```python
from build123d import *

# Parameters (mm, degrees)
SKETCH_2_R          = 7.1
SKETCH_2_R_2        = 6.1
EXTRUDE_1_DEPTH     = 2.2
SKETCH_2_3_R        = 9
SKETCH_2_3_R_2      = 7.1
EXTRUDE_2_DEPTH     = 4
EXTRUDE_3_DEPTH     = 4
SKETCH_4_W          = 46
SKETCH_4_H          = 28
SKETCH_4_W_2        = 38
SKETCH_4_H_2        = 21
EXTRUDE_4_DEPTH     = 4
EXTRUDE_1_2_DEPTH   = 4
DELETE_FACE_1_DEPTH = 4
FILLET_4_R          = 0.5
FILLET_5_R          = 0.4
FILLET_6_R          = 1


# Read off the part's stored shape, not the designer's step: 删除面1
with BuildPart() as part:
    # 草图2 → Extrude 1 (new body)
    with BuildSketch(Plane.XY):
        Circle(SKETCH_2_R)
        Circle(SKETCH_2_R_2, mode=Mode.SUBTRACT)
    extrude(amount=EXTRUDE_1_DEPTH)

    # 草图2<3> → 凸台-拉伸2 (add)
    with BuildSketch(Plane.XY):
        Circle(SKETCH_2_3_R)
        Circle(SKETCH_2_3_R_2, mode=Mode.SUBTRACT)
    extrude(amount=EXTRUDE_2_DEPTH)

    # 草图3 → 凸台-拉伸3 (add)
    with BuildSketch(Plane.XY):
        with BuildLine():
            Line((6, 6.708203932), (6, 9.5))
            Line((6, 9.5), (-6, 9.5))
            Line((-6, 9.5), (-6, 6.708203932))
            ThreePointArc((-6, 6.708203932), (0, 9), (6, 6.708203932))
        make_face()
        with BuildLine():
            Line((-6, -9.5), (6, -9.5))
            Line((6, -9.5), (6, -6.708203932))
            ThreePointArc((6, -6.708203932), (0, -9), (-6, -6.708203932))
            Line((-6, -6.708203932), (-6, -9.5))
        make_face()
    extrude(amount=EXTRUDE_3_DEPTH)



with BuildPart() as body_2:
    # 草图4 → 凸台-拉伸4 (new body)
    with BuildSketch(Plane.XY):
        with Locations((0, 1)):
            Rectangle(SKETCH_4_W, SKETCH_4_H)
        with Locations((0, 0.5)):
            Rectangle(SKETCH_4_W_2, SKETCH_4_H_2, mode=Mode.SUBTRACT)
    extrude(amount=EXTRUDE_4_DEPTH)


with BuildPart() as part_1:
    add(part.part)

    add(body_2.part)  # Extrude 1 2 merges body 2
    # 草图7 → Extrude 1 2 (add)
    with BuildSketch(Plane.XY):
        with BuildLine():
            ThreePointArc((19.19111663, -8.148610709), (15.188418529, -6.736776188), (10.944962783, -6.647601418))
            ThreePointArc((10.944962783, -6.647601418), (8.412688328, -7.06534444), (5.904962783, -7.611454086))
            Line((5.904962783, -7.611454086), (6.095037217, -8.388545914))
            ThreePointArc((6.095037217, -8.388545914), (8.562957594, -7.851104675), (11.055037217, -7.439992495))
            ThreePointArc((11.055037217, -7.439992495), (15.04515232, -7.523843398), (18.80888337, -8.851389291))
            Line((18.80888337, -8.851389291), (19.19111663, -8.148610709))
        make_face()
        with BuildLine():
            ThreePointArc((-18.80888337, -8.851389291), (-15.04515232, -7.523843398), (-11.055037217, -7.439992495))
            ThreePointArc((-11.055037217, -7.439992495), (-8.562957594, -7.851104675), (-6.095037217, -8.388545914))
            Line((-6.095037217, -8.388545914), (-5.904962783, -7.611454086))
            ThreePointArc((-5.904962783, -7.611454086), (-8.412688328, -7.06534444), (-10.944962783, -6.647601418))
            ThreePointArc((-10.944962783, -6.647601418), (-15.188418529, -6.736776188), (-19.19111663, -8.148610709))
            Line((-19.19111663, -8.148610709), (-18.80888337, -8.851389291))
        make_face()
        with BuildLine():
            ThreePointArc((-18.80888337, 7.148610709), (-15.04515232, 8.476156602), (-11.055037217, 8.560007505))
            ThreePointArc((-11.055037217, 8.560007505), (-8.562957594, 8.148895325), (-6.095037217, 7.611454086))
            Line((-6.095037217, 7.611454086), (-5.904962783, 8.388545914))
            ThreePointArc((-5.904962783, 8.388545914), (-8.412688328, 8.93465556), (-10.944962783, 9.352398582))
            ThreePointArc((-10.944962783, 9.352398582), (-15.188418529, 9.263223812), (-19.19111663, 7.851389291))
            Line((-19.19111663, 7.851389291), (-18.80888337, 7.148610709))
        make_face()
        with BuildLine():
            ThreePointArc((19.19111663, 7.851389291), (15.188418529, 9.263223812), (10.944962783, 9.352398582))
            ThreePointArc((10.944962783, 9.352398582), (8.412688328, 8.93465556), (5.904962783, 8.388545914))
            Line((5.904962783, 8.388545914), (6.095037217, 7.611454086))
            ThreePointArc((6.095037217, 7.611454086), (8.562957594, 8.148895325), (11.055037217, 8.560007505))
            ThreePointArc((11.055037217, 8.560007505), (15.04515232, 8.476156602), (18.80888337, 7.148610709))
            Line((18.80888337, 7.148610709), (19.19111663, 7.851389291))
        make_face()
    extrude(amount=EXTRUDE_1_2_DEPTH)

    # Delete Face 1 outline → Delete Face 1 (add)
    with BuildSketch(Plane.XY):
        with BuildLine():
            ThreePointArc((-19, 7.042506057), (-18.904671788, 7.095972847), (-18.80888337, 7.148610709))
            Line((-18.80888337, 7.148610709), (-19, 7.5))
            Line((-19, 7.5), (-19, 7.042506057))
        make_face()
        with BuildLine():
            Line((-6, 7.588108866), (-6, 8))
            Line((-6, 8), (-6.095037217, 7.611454086))
            ThreePointArc((-6.095037217, 7.611454086), (-6.047512851, 7.599804915), (-6, 7.588108866))
        make_face()
        with BuildLine():
            ThreePointArc((-19, -8.957493943), (-18.904671788, -8.904027153), (-18.80888337, -8.851389291))
            Line((-18.80888337, -8.851389291), (-19, -8.5))
            Line((-19, -8.5), (-19, -8.957493943))
        make_face()
        with BuildLine():
            Line((-6, -8.411891134), (-6, -8))
            Line((-6, -8), (-6.095037217, -8.388545914))
            ThreePointArc((-6.095037217, -8.388545914), (-6.047512851, -8.400195085), (-6, -8.411891134))
        make_face()
        with BuildLine():
            Line((6.095037217, 7.611454086), (6, 8))
            Line((6, 8), (6, 7.588108866))
            ThreePointArc((6, 7.588108866), (6.047512851, 7.599804915), (6.095037217, 7.611454086))
        make_face()
        with BuildLine():
            Line((19, 7.5), (18.80888337, 7.148610709))
            ThreePointArc((18.80888337, 7.148610709), (18.904671788, 7.095972847), (19, 7.042506057))
            Line((19, 7.042506057), (19, 7.5))
        make_face()
        with BuildLine():
            Line((6.095037217, -8.388545914), (6, -8))
            Line((6, -8), (6, -8.411891134))
            ThreePointArc((6, -8.411891134), (6.047512851, -8.400195085), (6.095037217, -8.388545914))
        make_face()
        with BuildLine():
            Line((19, -8.5), (18.80888337, -8.851389291))
            ThreePointArc((18.80888337, -8.851389291), (18.904671788, -8.904027153), (19, -8.957493943))
            Line((19, -8.957493943), (19, -8.5))
        make_face()
    extrude(amount=DELETE_FACE_1_DEPTH)

    # 圆角4
    fillet_4_edges = [part_1.edges().sort_by_distance(p)[0] for p in [
        (19, -8.046657496, 2),
        (6, -7.588305973, 2),
        (-19, -8.046657496, 2),
        (-6, -7.588305973, 2),
        (-6, 9.5, 2),
        (6, 9.5, 2),
        (6, 6.708203932, 2),
        (-6, 6.708203932, 2),
        (19, -8.957493943, 2),
        (-19, -8.957493943, 2),
        (-19, 7.042506057, 2),
        (19, 7.042506057, 2),
        (6, -6.708203932, 2),
        (-6, -6.708203932, 2),
        (-19, 7.953342504, 2),
        (19, 7.953342504, 2),
    ]]
    fillet(fillet_4_edges, radius=FILLET_4_R)

    # 圆角5
    fillet_5_edges = [part_1.edges().sort_by_distance(p)[0] for p in [
        (6, -8.411891134, 2),
        (-6, -8.411891134, 2),
        (-6, 7.588108866, 2),
        (6, 7.588108866, 2),
        (-6, -9.5, 2),
        (6, -9.5, 2),
        (-6, 8.411694027, 2),
        (-19, -10, 2),
        (19, -10, 2),
        (6, 8.411694027, 2),
    ]]
    fillet(fillet_5_edges, radius=FILLET_5_R)

    # 圆角6
    fillet_6_edges = [part_1.edges().sort_by_distance(p)[0] for p in [
        (19, 11, 2),
        (-19, 11, 2),
    ]]
    fillet(fillet_6_edges, radius=FILLET_6_R)


solid = part_1.part
```
Can you work these out from the model? Positions are in its coordinate system, mm. A direction names the side the tool comes from. Coordinates: 2 decimals unless noted, no trailing zeros. Loops run counter-clockwise (first coordinate to the right, second up) from the corner with the lowest first, then second, coordinate; pieces in that order, holes last.
Item 1: Which directions (+Z, -Z, +X, -X, +Y, -Y) give clear straight access to the entire face, cutting with the end or side of a thin tool? Please do faces 4 (the face through (-8.703, -7.824, 1.972)), 5 (the face through (-5, 4, 0)), 6 (the face through (2, 6, 2.2)).
Answers below:
face 4: +Z, -Z
face 5: -Z, +X, -X, +Y, -Y
face 6: +Z
Item 2: Suppose I cut it at C-C (z = 1.25). State how many separate pieces and enclosed holes the cut face has, then the cut area to 3 significant figures.
Answers below:
separate pieces: 1
enclosed holes: 5
area: 701 mm2
Item 3: Please list where these lines run through material, in increasing order: L1, parallel to Y at x = 0, z = 3.25; L2, parallel to Y at x = 0, z = 1.1; L3, parallel to X at y = 6.5, z = 0.9.
Answers below:
L1: y = -13 to -10, -9.5 to -7.1, 7.1 to 9.5, 11 to 15
L2: y = -13 to -10, -9.5 to -6.1, 6.1 to 9.5, 11 to 15
L3: x = -23 to -19, -6.22 to 6.22, 19 to 23
Item 4: Suppose I cut it at B-B (y = 2.25). Please give me the cut outline in (x, z).
Answers below:
outline: (-23, 0) - (-19, 0) - (-19, 4) - (-23, 4) - close; (-8.71, 0) - (-5.67, 0) - (-5.67, 2.2) - (-6.73, 2.2) - (-6.73, 4) - (-8.71, 4) - close; (5.67, 0) - (8.71, 0) - (8.71, 4) - (6.73, 4) - (6.73, 2.2) - (5.67, 2.2) - close; (19, 0) - (23, 0) - (23, 4) - (19, 4) - close
Item 5: Suppose I cut it at A-A (x = 0). Please give me the cut outline in (y, z), then the cut area to 3 significant figures.
Answers below:
outline: (-13, 0) - (-10, 0) - (-10, 4) - (-13, 4) - close; (-9.5, 0) - (-6.1, 0) - (-6.1, 2.2) - (-7.1, 2.2) - (-7.1, 4) - (-9.5, 4) - close; (6.1, 0) - (9.5, 0) - (9.5, 4) - (7.1, 4) - (7.1, 2.2) - (6.1, 2.2) - close; (11, 0) - (15, 0) - (15, 4) - (11, 4) - close
area: 51.6 mm2
Item 6: If we mould it in two halves opening along Y, with no side actions, what happens to faces 1 (the face through (0, 15, 2)), 2 (the face through (0, -10, 2)), 3 (the face through (23, 1, 2))? For each: released by +Y, released by -Y, zero draft, split by the parting line, or undercut.
Answers below:
face 1: released by +Y
face 2: undercut
face 3: zero draft
